Check sheet for the drawn part. Datum: minimum x, y, z corner. Units: mm. A direction names the side the tool comes from. Give positions to 0.01 mm unless a question says otherwise; leave off trailing zeros. Write each loop counter-clockwise with the first axis right and the second up, starting at its lowest first coordinate (ties: lowest second). Pieces come first, ordered by that corner, then holes. Notation, with made-up numbers: (19, 9.5) - (52, 9.5) arc R18 cw to (52, 17.5) - close; hole circle Ø8 at (76.25, -27). An arc over 180 degrees is marked (long way). One line per question, with ' | ' between items. Start each with the question number.
Q1. Thickness scan on L1, parallel to X at y = 4, z = 5.5; L2, parallel to Z at x = 2.75, y = 12.5 (1 decimal); L3, parallel to Y at x = 14.25, z = 23. Record the ranges inside material, lowest first. Write a range as [from, to].
Q2. Set-up check for the marked faces 5, 6 and 7: record each of +Z, -Z, +X, -X, +Y, -Y from which the full face is reachable in a straight line by a thin tool's end or side.
Q3. Section check A-A on z = 12. Record the boundary of the cut face in (x, y).
Q4. Gauge pin test, flat ends, axial feed: P1, Ø5, axis at x = 13.5, y = 18.5, coming from the -Z side (3 decimals); P2, Ø4, axis at x = 6, z = 24, coming from the +Y side. Record the tip position at first contact, or that the pin passes through.
Q5. Release check for a two-part mould opening along X. For the marked faces 1, 2, 3 and 4 record: +X half, -X half, draft (parallel to the pull), parting line (faces both ways), or undercut.
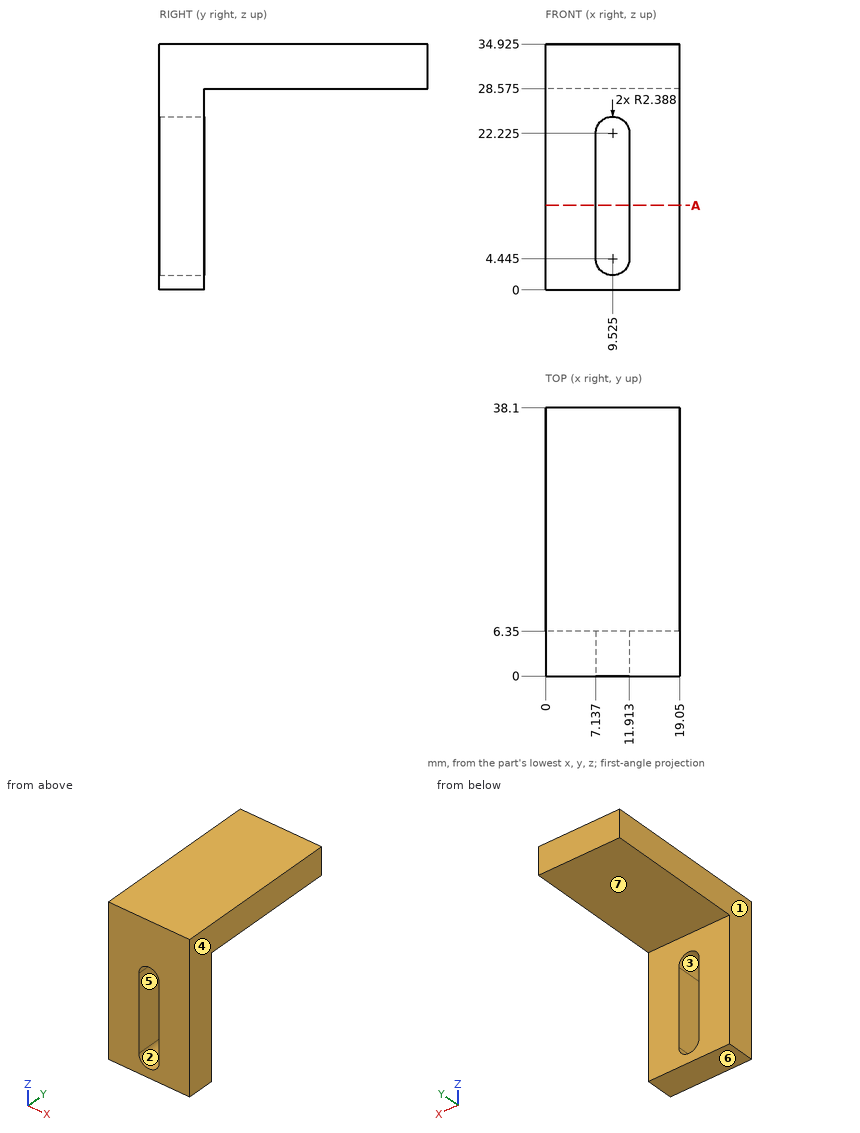
Working result:
1) L1: x = [0, 7.14], [11.91, 19.05] | L2: z = [28.6, 34.9] | L3: y = [0, 6.35]
2) face 5: +Y, -Y | face 6: -Z, +X, -X, +Y, -Y | face 7: -Z, +X, -X, +Y
3) outline: (0, 0) - (7.14, 0) - (7.14, 6.35) - (0, 6.35) - close; (11.91, 0) - (19.05, 0) - (19.05, 6.35) - (11.91, 6.35) - close
4) P1: stops at z = 28.575 | P2: stops at y = 6.35
5) face 1: -X half | face 2: undercut | face 3: undercut | face 4: +X half
